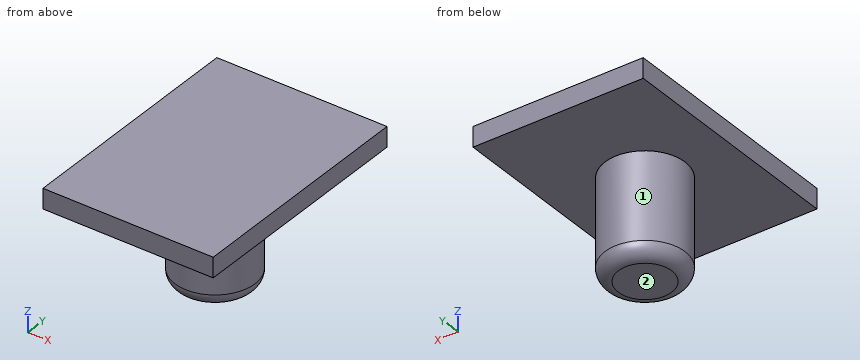
Autodesk Inventor part; units mm, degrees
ref_plane "YZ Plane" through (0, 0, 0) normal (1, 0, 0) x (0, 1, 0)
ref_plane "XZ Plane" through (0, 0, 0) normal (0, 1, 0) x (-1, 0, 0)
ref_plane "XY Plane" through (0, 0, 0) normal (0, 0, 1) x (1, 0, 0)
sketch "Sketch1" plane through (0, 0, 0) normal (0, 0, 1) x (1, 0, 0)
  line L0 (2.554, -3.555) -> (-2.554, -3.555)
  line L1 (-2.554, -3.555) -> (-2.554, 3.555)
  line L2 (-2.554, 3.555) -> (2.554, 3.555)
  line L3 (2.554, 3.555) -> (2.554, -3.555)
  line L4 (2.554, -3.555) -> (-2.554, 3.555) construction
  line L5 (-2.554, -3.555) -> (2.554, 3.555) construction
  point P0 (0, 0)
  dimension "d0" = 5.108
  dimension "d1" = 7.11
sketch "Sketch2" plane through (0, 0, 0) normal (0, 0, 1) x (1, 0, 0)
  circle A0 centre (0, 0) radius 1.2
  dimension "d2" = 2.4
extrude "Extrusion1" add sketch "Sketch1" along normal blind 0.6
extrude "Extrusion2" add sketch "Sketch2" against normal blind 3
fillet "Fillet1" radius 0.4 1 edges at (-1.2, 0, -3)
properties part number "tombol"
Check sheet for the modelled part. Datum: model origin and axes. Units: mm. Face numbers are marked on the shaded views. A direction names the side the tool comes from. Round coordinates to 2 decimals unless told otherwise and drop trailing zeros. Order: outer loops, then holes, each group sorted by start corner. A loop starts at its lowest first (then second) coordinate and runs counter-clockwise, first axis right, second up. Notation, with made-up numbers: M -13.5,6 L 5.5,6 A21 ccw 5.5,12 Z; hole C 18.25,20.25 d10. An arc over 180 degrees is marked long. One line per item, written item: value. Start each with the question number.
1. Section check B-B on x = 0. Enter the section's corners in (y, z) (3 decimals), and give its area (3 significant figures).
2. Access from +Z, -Z, +X, -X, +Y, -Y to the whole of each face (thin tool, end or side, straight path). Record for the marked faces 1 and 2.
3. Section check A-A on y = 0. Enter the section's corners in (x, z).
4. Section check C-C on z = -1.65. Enter the section's corners in (x, y), and give its area (3 significant figures).
5. Section check D-D on x = -1.45. Enter the section's corners in (y, z) (3 decimals).
6. Scan lines: line 1 along Z through (x, y) = (1.3, 0.75); line 2 along Y through (x, z) = (-0.05, -1.7); line 3 along Z through (x, y) = (-0.8, -0.25). Record each from-to range of solid material in increasing order.
Results found:
1. outline: M -3.555,0 L -1.2,0 L -1.2,-2.6 A0.4 ccw -0.8,-3 L 0.8,-3 A0.4 ccw 1.2,-2.6 L 1.2,0 L 3.555,0 L 3.555,0.6 L -3.555,0.6 Z
1. area: 11.4 mm^2
2. face 1: -Z
2. face 2: -Z, +X, -X, +Y, -Y
3. outline: M -2.55,0 L -1.2,0 L -1.2,-2.6 A0.4 ccw -0.8,-3 L 0.8,-3 A0.4 ccw 1.2,-2.6 L 1.2,0 L 2.55,0 L 2.55,0.6 L -2.55,0.6 Z
4. outline: C 0,0 d2.4
4. area: 4.52 mm^2
5. outline: M -3.555,0 L 3.555,0 L 3.555,0.6 L -3.555,0.6 Z
6. line 1: 0 to 0.6
6. line 2: -1.2 to 1.2
6. line 3: -3 to 0.6
